Design review of the part shown in the three views and the two pictorial views. Dimensions are in mm from the part's minimum x, y and z. Coordinates: 2 decimals unless noted, no trailing zeros. Loops run counter-clockwise (first coordinate to the right, second up) from the corner with the lowest first, then second, coordinate; pieces in that order, holes last.
Q1. Draft analysis for pull direction X (two halves, no side actions). For the marked faces 1, 2, 3 and 4, state which applies: released by +X, released by -X, zero draft, split by the parting line, or undercut.
Q2. For P1, Ø5, axis at x = 29, z = 7.5, coming from the -Y side; P2, Ø1, axis at x = 51.5, y = 28, coming from the -Z side; P3, Ø3, axis at x = 52.5, z = 3.5, coming from the +Y side, all flat-tipped, find the tip position at first contact; note any pin that passes through.
Q3. Add section C-C on y = 43. Give the boundary of the cut face in (x, z), and give its area (3 significant figures).
Q4. Add section A-A on z = 7.5. Give the boundary of the cut face in (x, y) (1 decimal).
Q5. Add section B-B on z = 11.5. Give the boundary of the cut face in (x, y) (1 decimal), and give its area (3 significant figures).
Q6. Wall thickness on probe 1 along Y at (x, z) = (50, 9); probe 2 along Y at (x, z) = (10, 7); probe 3 along Y at (x, z) = (50, 5.75): over which ranges is each line inside the solid? List them lowest first.
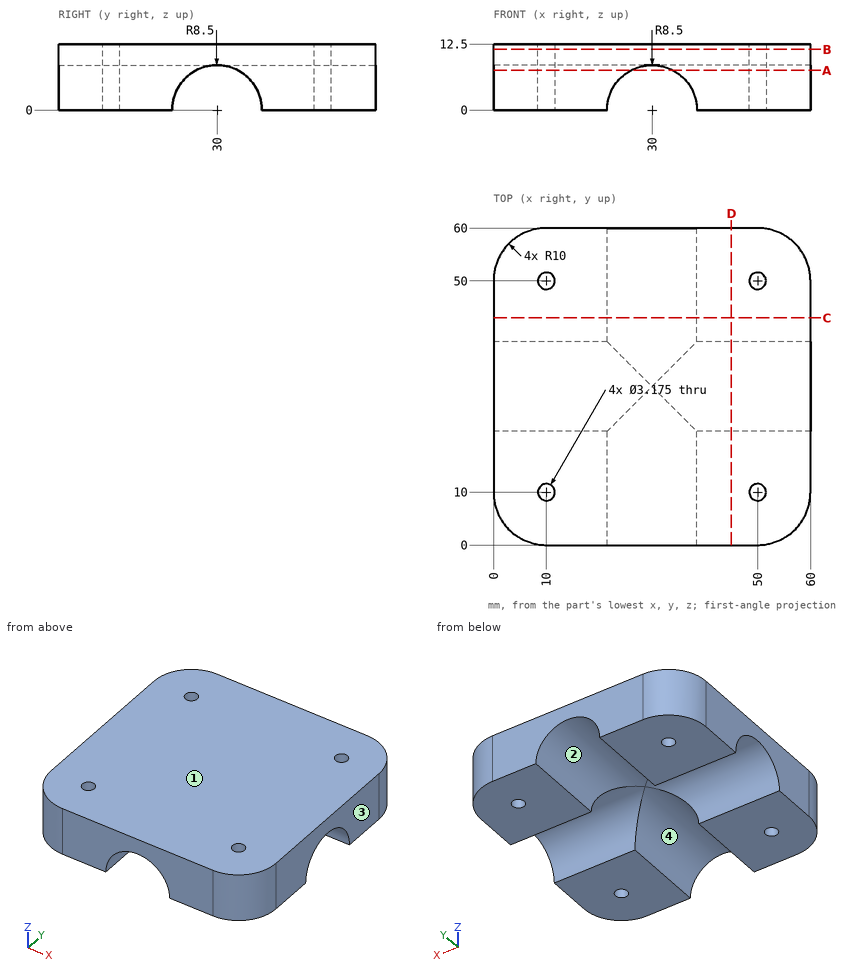
Entries:
1. face 1: zero draft
1. face 2: undercut
1. face 3: released by +X
1. face 4: undercut
2. P1: stops at y = 0
2. P2: stops at z = 8.12
2. P3: stops at y = 59.95
3. outline: (0, 0) - (21.5, 0) arc R8.5 cw to (38.5, 0) - (60, 0) - (60, 12.5) - (0, 12.5) - close
3. area: 637 mm2
4. outline: (0, 10) arc R10 ccw to (10, 0) - (26, 0) - (26, 26) - (0, 26) - close; (0, 34) - (26, 34) - (26, 60) - (10, 60) arc R10 ccw to (0, 50) - close; (34, 0) - (50, 0) arc R10 ccw to (60, 10) - (60, 26) - (34, 26) - close; (34, 34) - (60, 34) - (60, 50) arc R10 ccw to (50, 60) - (34, 60) - close; hole circle Ø3.2 at (10, 10); hole circle Ø3.2 at (10, 50); hole circle Ø3.2 at (50, 10); hole circle Ø3.2 at (50, 50)
5. outline: (0, 10) arc R10 ccw to (10, 0) - (50, 0) arc R10 ccw to (60, 10) - (60, 50) arc R10 ccw to (50, 60) - (10, 60) arc R10 ccw to (0, 50) - close; hole circle Ø3.2 at (10, 10); hole circle Ø3.2 at (10, 50); hole circle Ø3.2 at (50, 10); hole circle Ø3.2 at (50, 50)
5. area: 3,480 mm2
6. probe 1: y = 0 to 8.41, 11.59 to 48.41, 51.59 to 60
6. probe 2: y = 0 to 8.41, 11.59 to 25.18, 34.82 to 48.41, 51.59 to 60
6. probe 3: y = 0 to 8.41, 11.59 to 23.74, 36.26 to 48.41, 51.59 to 60
